Work out the finished part from the listing and answer in its coordinate system (mm). A direction names the side the tool comes from. Give positions to 0.01 mm unless a question says otherwise; leave off trailing zeros. Loops run counter-clockwise (first coordinate to the right, second up) from the corner with the lowest first, then second, coordinate; pieces in that order, holes last.
```python
from build123d import *

# Parameters (mm, degrees)
CUT_EXTRUDE1_DEPTH = 1.04


with BuildPart() as part:
    # Sketch1 → Revolve1 (revolve)
    with BuildSketch(Plane(origin=(0, 0, 0), x_dir=(1, 0, 0), z_dir=(0, 1, 0))):
        with BuildLine():
            Line((0, 0), (9.65, 0))
            Line((9.65, 0), (9.65, 1.5))
            Line((9.65, 1.5), (1.65, 1.5))
            Line((1.65, 1.5), (1.65, 2.85))
            Line((1.65, 2.85), (1.5, 2.85))
            ThreePointArc((1.5, 2.85), (0.439339828, 2.410660172), (0, 1.35))
            Line((0, 1.35), (0, 0))
        make_face()
    revolve(axis=Axis((0, 0, 0), (-1, 0, 0)))

    # Sketch2 → Cut-Extrude1 (cut)
    with BuildSketch(Plane.ZY):
        Polygon((1.154700538, 0), (0.577350269, 1), (-0.577350269, 1), (-1.154700538, 0), (-0.577350269, -1), (0.577350269, -1), align=None)
    extrude(amount=-CUT_EXTRUDE1_DEPTH, mode=Mode.SUBTRACT)


solid = part.part
```
Q1. Which of the six approach directions +Z, -Z, +X, -X, +Y, -Y give full straight-line access (tool end or side, diameter ignored) to faces 1 (the face through (1.65, 1.2, 1.2)), 2 (the face through (1.04, 0, 0))?
Q2. Given pin 1 (1.5 mm diameter, centred on x = 8, z = 1.5, fed in from -Y); pin 2 (1.1 mm diameter, centred on x = 0.5, z = 0, fed in from -Y); pin 3 (1.1 mm diameter, centred on x = 0.5, z = 0, fed in from +Y), each flat-ended and moving along its own axis, determine where each tip first touches the part or whether it passes through.
Q3. Determine the mould class of faces 3 (the face through (0.51, 0.49, 0.87)), 4 (the face through (9.65, 0, 0)), 5 (the face through (5.59, -0.07, 1.5)) for opening direction Z: +Z half, -Z half, draft (parallel to the pull), parting line (faces both ways), or undercut.
Q4. Consider line 1 along X through (y, z) = (0.45, 0.1); line 2 along Y through (x, z) = (5, -0.1); line 3 along X through (y, z) = (2.5, 0.5). Determine where each line is inside the solid, lowest interval first.
Q5. Section A-A on x = 9 is taken. Give the vertices of the cut face in (y, z).
Check result:
1. face 1: +X
1. face 2: -X
2. pin 1: stops at y = -1.3
2. pin 2: stops at y = -2.78
2. pin 3: stops at y = 2.78
3. face 3: undercut
3. face 4: draft
3. face 5: parting line
4. line 1: x = 1.04 to 9.65
4. line 2: y = -1.5 to 1.5
4. line 3: x = 0.6 to 1.65
5. outline: circle Ø3 at (0, 0)
